Part model, mm, in its own coordinate system. Face numbers are marked on the shaded views. A direction names the side the tool comes from. Give positions to 0.01 mm unless a question says otherwise; leave off trailing zeros. Order: outer loops, then holes, each group sorted by start corner. A loop starts at its lowest first (then second) coordinate and runs counter-clockwise, first axis right, second up. Notation, with made-up numbers: (-32, 0.25) - (22, 0.25) arc R12 ccw to (22, 11.25) - close; hole circle Ø10 at (-4.75, 61). An arc over 180 degrees is marked (long way). One line per item, written item: value.
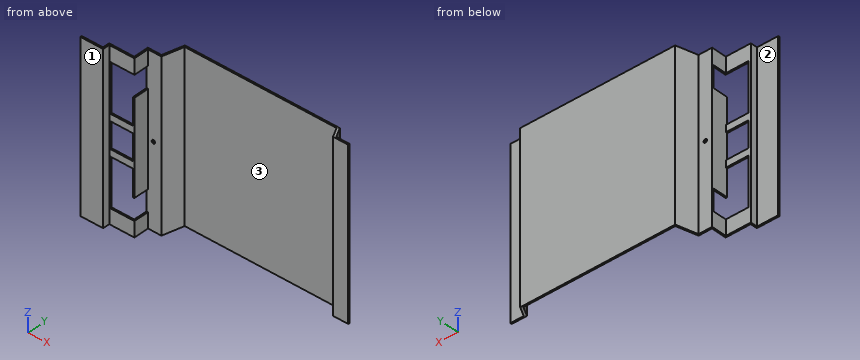
```python
from build123d import *

# Parameters (mm, degrees)
DODANIE_WYCI_GNI_CIE1_DEPTH = 109
SZKIC2_W                    = 30
SZKIC2_H                    = 63
SZKIC2_H_2                  = 34
WYTNIJ_WYCI_GNI_CIE1_DEPTH  = 2
OTW_R_POD_RUB_M41_D         = 4.5
OTW_R_POD_RUB_M41_DEPTH     = 2
SZKIC5_W                    = 28
SZKIC5_H                    = 20
WYTNIJ_WYCI_GNI_CIE2_DEPTH  = 3


with BuildPart() as part:
    # Szkic1 → Dodanie-wyciągnięcie1 (new body, symmetric)
    with BuildSketch(Plane.XY):
        Polygon((0, 0), (0, 2), (28, 2), (28, 11), (61, 11), (61, 31), (79, 31), (85.419782204, 58), (289.419782204, 58), (296.419782204, 45), (314, 45), (314, 43), (294, 43), (287, 56), (87, 56), (80.580217796, 29), (63, 29), (63, 9), (30, 9), (30, 0), align=None)
    extrude(amount=DODANIE_WYCI_GNI_CIE1_DEPTH, both=True)

    # Szkic2 → Wytnij-wyciągnięcie1 (cut)
    with BuildSketch(Plane(origin=(0, 11, 0), x_dir=(1, 0, 0), z_dir=(0, 1, 0))):
        with Locations((46, 57.5)):
            Rectangle(SZKIC2_W, SZKIC2_H)
        with Locations((46, 0)):
            Rectangle(SZKIC2_W, SZKIC2_H_2)
        with Locations((46, -57.5)):
            Rectangle(SZKIC2_W, SZKIC2_H)
    extrude(amount=-WYTNIJ_WYCI_GNI_CIE1_DEPTH, mode=Mode.SUBTRACT)

    # Otwór pod śrubę M41
    with Locations(Plane(origin=(70, 31, 0), x_dir=(0, 0, 1), z_dir=(0, 1, 0))):
        with Locations((0, 0)):
            Hole(OTW_R_POD_RUB_M41_D / 2, depth=OTW_R_POD_RUB_M41_DEPTH)

    # Szkic5 → Wytnij-wyciągnięcie2 (cut)
    with BuildSketch(Plane.ZY.offset(-61)):
        with Locations((-75, 19)):
            Rectangle(SZKIC5_W, SZKIC5_H)
        with Locations((75, 19)):
            Rectangle(SZKIC5_W, SZKIC5_H)
    extrude(amount=-WYTNIJ_WYCI_GNI_CIE2_DEPTH, mode=Mode.SUBTRACT)


solid = part.part
```
1) Slice it at A-A on z = 46. Write the cut outline in (x, y).
Answer:
outline: (0, 0) - (30, 0) - (30, 9) - (31, 9) - (31, 11) - (28, 11) - (28, 2) - (0, 2) - close; (61, 9) - (63, 9) - (63, 29) - (80.58, 29) - (87, 56) - (287, 56) - (294, 43) - (314, 43) - (314, 45) - (296.42, 45) - (289.42, 58) - (85.42, 58) - (79, 31) - (61, 31) - close
2) Slice it at D-D on x = 170. Write the cut outline in (y, z).
Answer:
outline: (56, -109) - (58, -109) - (58, 109) - (56, 109) - close
3) Drop flat-ended pins along their axis: P1, Ø10, axis at x = 44, z = 16, coming from the +Y side; P2, Ø10, axis at y = 21.5, z = -20, coming from the +X side; P3, Ø6, axis at y = 6.5, z = 11, coming from the -X side; P4, Ø5, axis at x = 51, y = 13, coming from the -Z side. Give the stop position or say it passes through.
Answer:
P1: stops at y = 11
P2: stops at x = 63
P3: stops at x = 28
P4: stops at z = -109
4) Slice it at C-C on z = -79. Write the cut outline in (x, y).
Answer:
outline: (0, 0) - (30, 0) - (30, 9) - (31, 9) - (31, 11) - (28, 11) - (28, 2) - (0, 2) - close; (61, 29) - (80.58, 29) - (87, 56) - (287, 56) - (294, 43) - (314, 43) - (314, 45) - (296.42, 45) - (289.42, 58) - (85.42, 58) - (79, 31) - (61, 31) - close
5) Wall check: line 1 along Y through (x, z) = (109, 10); line 2 along X through (y, z) = (4, 36); line 3 along X through (y, z) = (30.35, 0). Give the ranges that are in metal, low to high. Write a range as [from, to].
Answer:
line 1: y = [56, 58]
line 2: x = [28, 30]
line 3: x = [61, 67.75], [72.25, 80.9]
6) Slice it at B-B on y = 24. Write the cut outline in (x, z).
Answer:
outline: (61, -109) - (63, -109) - (63, -89) - (61, -89) - close; (61, -61) - (63, -61) - (63, 61) - (61, 61) - close; (61, 89) - (63, 89) - (63, 109) - (61, 109) - close
7) Which spindle directions (+Z, -Z, +X, -X, +Y, -Y) get a long thin tool onto all of the face, cutting with end or side? Do the marked faces 1, 2 and 3. Say none if no direction does.
Answer:
face 1: +Z, -Z, +X, -X, -Y
face 2: +Z, -Z, -X, +Y
face 3: +Z, -Z, -Y
